from build123d import *

# Parameters (mm, degrees)
F1_R     = 30
F1_R_2   = 82.5
F3_DEPTH = 20
F4_R     = 82.5
F4_R_2   = 30
F5_DEPTH = 20


with BuildPart() as f2:
    # F2: sweep along a path in F0
    with BuildLine(Plane.XY) as f2_path:
        Line((0, 0), (350, 0))
        ThreePointArc((350, 0), (456.066017178, -43.933982822), (500, -150))
        Line((500, -150), (500, -850))
        ThreePointArc((500, -850), (543.933982822, -956.066017178), (650, -1000))
        Line((650, -1000), (1037, -1000))
    # F1 (on Right) → F2 (sweep)
    with BuildSketch(Plane.YZ):
        Circle(F1_R)
    sweep(path=f2_path.line)

    # F1 (on Right) → F3 (join)
    with BuildSketch(Plane.YZ):
        Circle(F1_R_2)
        Circle(F1_R, mode=Mode.SUBTRACT)
    extrude(amount=F3_DEPTH)

    # F4 (on face) → F5 (join)
    with BuildSketch(Plane.YZ.offset(1037)):
        with Locations((-1000, 0)):
            Circle(F4_R)
        with Locations((-1000, 0)):
            Circle(F4_R_2, mode=Mode.SUBTRACT)
    extrude(amount=-F5_DEPTH)


solid = f2.part
Source: CAD feature listing. Evaluate the final solid. Frame: model axes, mm. Coordinates: 2 decimals unless noted, no trailing zeros. Loops run counter-clockwise (first coordinate to the right, second up) from the corner with the lowest first, then second, coordinate; pieces in that order, holes last. Notation, with made-up numbers: M 59,62 L 64,62 A20 ccw 64,90 Z; hole C 68,74 d2. An arc over 180 degrees is marked long. Answer in a Markdown table with one row per item.
Q1. Section A-A on z = 0. Return the cut outline in (x, y).
Answers below:
| item | result |
|---|---|
| outline | M 0,-82.5 L 20,-82.5 L 20,-30 L 350,-30 A120 cw 470,-150 L 470,-850 A180 ccw 650,-1030 L 1017,-1030 L 1017,-1082.5 L 1037,-1082.5 L 1037,-917.5 L 1017,-917.5 L 1017,-970 L 650,-970 A120 cw 530,-850 L 530,-150 A180 ccw 350,30 L 20,30 L 20,82.5 L 0,82.5 Z |
Q2. Ray query, probe 1 along X at (y, z) = (-424, 1.5); probe 2 along X at (y, z) = (-1030.5, -38.5); probe 3 along Y at (x, z) = (102, 13). Return the intervals inside material, ascending. Write a range as from..to.
Answers below:
| item | result |
|---|---|
| probe 1 | x = 470.04..529.96 |
| probe 2 | x = 1017..1037 |
| probe 3 | y = -27.04..27.04 |
Q3. Draft query along X for faces 1 (the flat face through (0, -1, 1)), 2 (the flat face through (1017, -1001, -36)), 3 (the flat face through (1037, -1001, 1)), 4 (the cylindrical face through (9.86, -17.88, -80.54)). Return one class per face: pulls with the +X half, pulls with the -X half, needs draft (parallel to the pull), parting line crosses it, or undercut.
Answers below:
| item | result |
|---|---|
| face 1 | pulls with the -X half |
| face 2 | undercut |
| face 3 | pulls with the +X half |
| face 4 | needs draft |
Q4. Section C-C on y = -734.5. Return the cut outline in (x, z), plus the area to 3 significant figures.
Answers below:
| item | result |
|---|---|
| outline | C 500,0 d60 |
| area | 2,830 mm^2 |
Q5. Section D-D on x = 885. Return the cut outline in (y, z), plus the area to 3 significant figures.
Answers below:
| item | result |
|---|---|
| outline | C -1000,0 d60 |
| area | 2,830 mm^2 |
Q6. Section B-B on z = 68. Return the cut outline in (x, y).
Answers below:
| item | result |
|---|---|
| outline | M 0,-46.71 L 20,-46.71 L 20,46.71 L 0,46.71 Z; M 1017,-1046.71 L 1037,-1046.71 L 1037,-953.29 L 1017,-953.29 Z |
Q7. First-contact query: pin 1 (5 mm diameter, centred on y = -378, z = -18, fed in from +X); pin 2 (2 mm diameter, centred on y = -205, z = 1, fed in from +X); pin 3 (4 mm diameter, centred on y = -581.5, z = -20, fed in from -X). Flat tips, straight axial feed; report the tip coordinate or a pass-through.
Answers below:
| item | result |
|---|---|
| pin 1 | stops at x = 525.69 |
| pin 2 | stops at x = 530 |
| pin 3 | stops at x = 476 |
